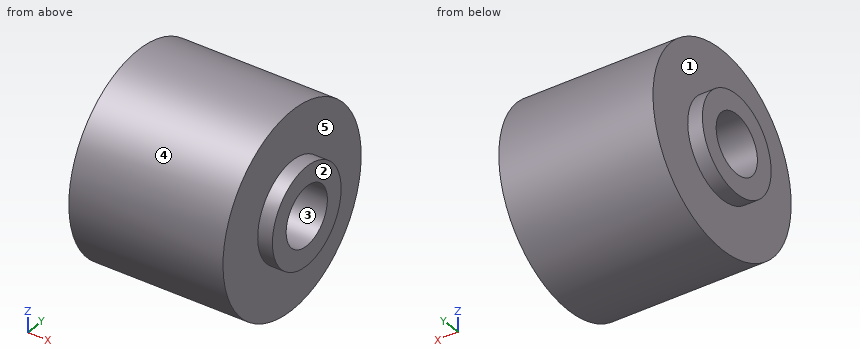
from build123d import *

# Parameters (mm, degrees)
SZKIC1_W   = 31.5
SZKIC1_H   = 14.1
SZKIC1_W_2 = 3
SZKIC1_H_2 = 4


with BuildPart() as part:
    # Szkic1 → Obrót1 (revolve)
    with BuildSketch(Plane.XY, mode=Mode.PRIVATE) as obr_t1_sk:
        with Locations((0, 13.05)):
            Rectangle(SZKIC1_W, SZKIC1_H)
        with Locations((-17.25, 8)):
            Rectangle(SZKIC1_W_2, SZKIC1_H_2)
        with Locations((17.25, 8)):
            Rectangle(SZKIC1_W_2, SZKIC1_H_2)
    revolve(obr_t1_sk.sketch.rotate(Axis((0, 0, 0), (-1, 0, 0)), 90), axis=Axis((0, 0, 0), (-1, 0, 0)))


solid = part.part
Work out the finished part from the listing and answer in its coordinate system (mm). Face numbers are marked on the shaded views. A direction names the side the tool comes from. Round coordinates to 2 decimals unless told otherwise and drop trailing zeros. Order: outer loops, then holes, each group sorted by start corner. A loop starts at its lowest first (then second) coordinate and runs counter-clockwise, first axis right, second up. Notation, with made-up numbers: M -27,-25.75 L 20,-25.75 A28 cw 20,7.25 Z; hole C -20.75,-15 d1. An arc over 180 degrees is marked long. One line per item, written item: value.
Q1. Straight lines are drawn through the part: line 1 (Y direction, x = 10, z = 0); line 2 (Y direction, x = 15.5, z = 2.5); line 3 (X direction, y = -12.5, z = 15.5). For each, find the intervals that lie inside material, in ascending order.
Derived:
line 1: -20.1 to -6, 6 to 20.1
line 2: -19.94 to -5.45, 5.45 to 19.94
line 3: -15.75 to 15.75
Q2. Find section D-D on y = -12. Write down the section's boundary in (x, z).
Derived:
outline: M -15.75,-16.12 L 15.75,-16.12 L 15.75,16.12 L -15.75,16.12 Z
Q3. Flat-ended cylindrical pins translate along their axes: pin 1 (1.5 mm diameter, centred on x = 12, z = 7.5, fed in from +Y); pin 2 (6 mm diameter, centred on x = -9.5, z = 14, fed in from -Y); pin 3 (3 mm diameter, centred on x = 8.5, z = -6, fed in from -Y). Find the tip coordinate at first contact, or state that the pin passes through.
Derived:
pin 1: y = 18.93
pin 2: y = -16.82
pin 3: y = -19.59
Q4. Determine the mould class of the marked faces 3, 4 and 5 for opening direction Z: released by +Z, released by -Z, zero draft, split by the parting line, or undercut.
Derived:
face 3: undercut
face 4: split by the parting line
face 5: zero draft
Q5. Find section A-A on y = 0. Write down the section's boundary in (x, z).
Derived:
outline: M -18.75,-10 L -15.75,-10 L -15.75,-20.1 L 15.75,-20.1 L 15.75,-10 L 18.75,-10 L 18.75,-6 L -18.75,-6 Z; M -18.75,6 L 18.75,6 L 18.75,10 L 15.75,10 L 15.75,20.1 L -15.75,20.1 L -15.75,10 L -18.75,10 Z
Q6. Find section C-C on x = -3. Write down the section's boundary in (y, z).
Derived:
outline: C 0,0 d40.2; hole C 0,0 d12
Q7. For the marked faces 1 and 2, determine the directions among +Z, -Z, +X, -X, +Y, -Y from which every point of the face is accessible in a straight line to the end or side of a thin tool.
Derived:
face 1: -X
face 2: +Z, -Z, +X, +Y, -Y
